Input: dimensioned drawing with shaded views. Units: mm. Origin: part minimum x, y, z. A direction names the side the tool comes from. Give positions to 0.01 mm unless a question says otherwise; leave off trailing zeros. Write each loop counter-clockwise with the first axis right and the second up, starting at its lowest first coordinate (ties: lowest second). Pieces come first, ordered by that corner, then holes. Notation, with made-up numbers: (-13, 12) -> (45, 12) arc R11 ccw to (45, 26) -> close; hole circle Ø9 at (-29.75, -14.5). An arc over 180 degrees is marked (long way). Return JSON: item names as keys, results as strings. Group by question number.
Item 1: Line query: line 1 (X direction, y = 49.5, z = 83.5); line 2 (Z direction, x = 72.5, y = 13); line 3 (Z direction, x = 91, y = 6.5). Output: solid intervals per line, ascending. Write a range as [from, to].
Item 2: Pin query (flat end, axial travel): P1, Ø2, axis at x = 52, y = 26, coming from the +Z side. Return the tip coordinate at first contact, or that it passes through.
Item 3: Section D-D, the plane x = 50. Return loops of the section in (y, z).
Item 4: Set-up query: the marked faces 4 and 5. Return all of +Z, -Z, +X, -X, +Y, -Y with unobstructed straight access to the full face (end or side cutting, diameter ignored); none if empty.
Item 5: Section C-C, the plane x = 17. Return loops of the section in (y, z), then the cut area to 3 significant figures.
Item 6: Mould query, pull axis X, two halves, no side actions, for the marked faces 1, 2 and 3. Classes: released by +X, released by -X, zero draft, split by the parting line, or undercut.
Item 7: Section A-A, the plane z = 78.5. Return loops of the section in (x, y).
Item 8: Section B-B, the plane y = 42. Return loops of the section in (x, z), then the cut area to 3 significant figures.
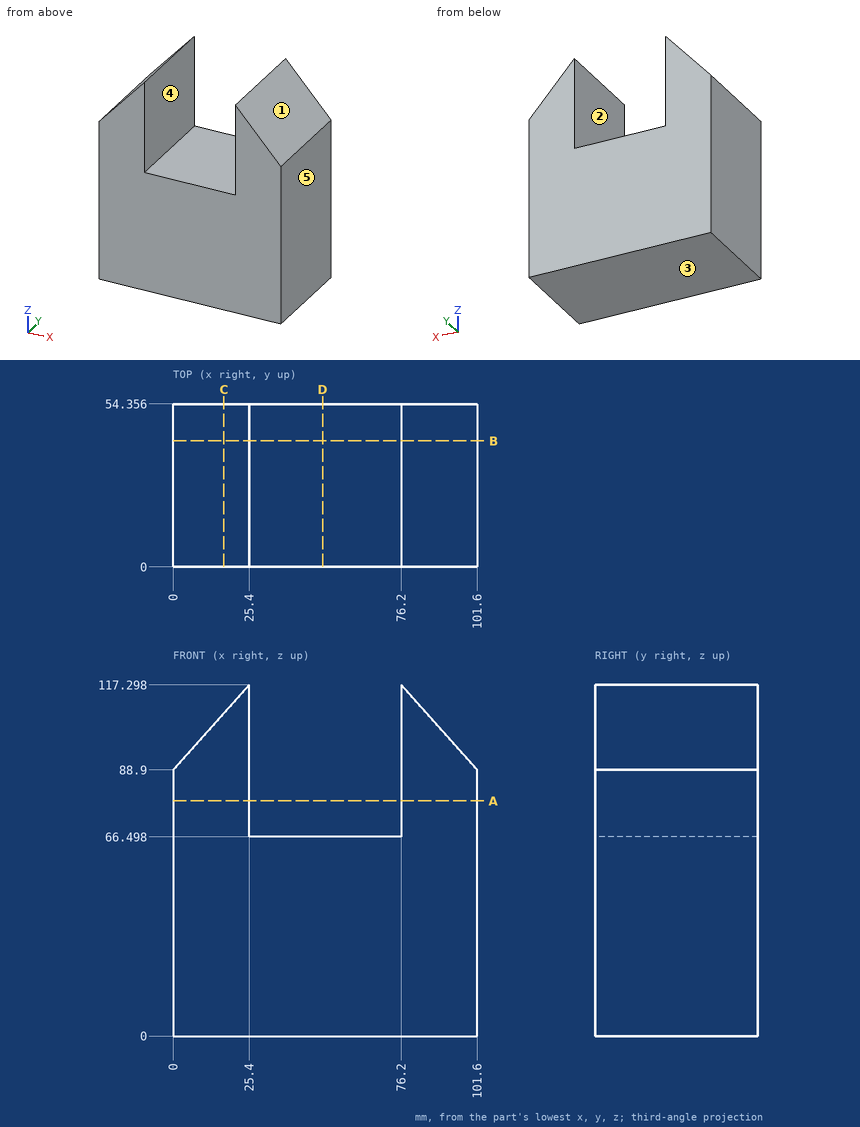
Answer below:
{
 "1": {"line 1": "x = [0, 25.4], [76.2, 101.6]", "line 2": "z = [0, 66.5]", "line 3": "z = [0, 100.75]"},
 "2": {"P1": "stops at z = 66.5"},
 "3": {"outline": "(0, 0) -> (54.36, 0) -> (54.36, 66.5) -> (0, 66.5) -> close"},
 "4": {"face 4": "+Z, +Y, -Y", "face 5": "+Z, -Z, +X, +Y, -Y"},
 "5": {"outline": "(0, 0) -> (54.36, 0) -> (54.36, 107.91) -> (0, 107.91) -> close", "area": "5,870 mm2"},
 "6": {"face 1": "released by +X", "face 2": "undercut", "face 3": "zero draft"},
 "7": {"outline": "(0, 0) -> (25.4, 0) -> (25.4, 54.36) -> (0, 54.36) -> close; (76.2, 0) -> (101.6, 0) -> (101.6, 54.36) -> (76.2, 54.36) -> close"},
 "8": {"outline": "(0, 0) -> (101.6, 0) -> (101.6, 88.9) -> (76.2, 117.3) -> (76.2, 66.5) -> (25.4, 66.5) -> (25.4, 117.3) -> (0, 88.9) -> close", "area": "8,620 mm2"}
}
